Autodesk Inventor part; units mm, degrees
ref_plane "YZ Plane" through (0, 0, 0) normal (1, 0, 0) x (0, 1, 0)
ref_plane "XZ Plane" through (0, 0, 0) normal (0, 1, 0) x (-1, 0, 0)
ref_plane "XY Plane" through (0, 0, 0) normal (0, 0, 1) x (1, 0, 0)
sketch "Sketch1" plane through (0, 0, 0) normal (0, 1, 0) x (-1, 0, 0)
  line L0 (12.7, -15.875) -> (12.7, -12.7) construction
  line L1 (12.7, -12.7) -> (15.875, -10.8669) construction
  line L2 (15.875, -10.8669) -> (15.875, -7.9375) construction
  line L3 (15.875, -7.9375) -> (6.35, -7.9375) construction
  line L4 (6.35, -7.9375) -> (6.35, -3.175) construction
  line L5 (6.35, -3.175) -> (3.175, -3.175) construction
  line L6 (3.175, -3.175) -> (3.175, -6.35) construction
  line L7 (3.175, -6.35) -> (4.7625, -7.2665) construction
  line L8 (4.7625, -7.2665) -> (4.7625, -7.9375) construction
  line L9 (4.7625, -7.9375) -> (-4.7625, -7.9375) construction
  line L10 (-4.7625, -7.9375) -> (-4.7625, -7.2665) construction
  line L11 (-4.7625, -7.2665) -> (-3.175, -6.35) construction
  line L12 (-3.175, -6.35) -> (-3.175, -3.175) construction
  line L13 (-3.175, -3.175) -> (-6.35, -3.175) construction
  line L14 (-6.35, -3.175) -> (-6.35, -7.9375) construction
  line L15 (-6.35, -7.9375) -> (-15.875, -7.9375) construction
  line L16 (-15.875, -7.9375) -> (-15.875, -10.8669) construction
  line L17 (-15.875, -10.8669) -> (-12.7, -12.7) construction
  line L18 (-12.7, -12.7) -> (-12.7, -15.875) construction
  line L19 (-25.4, -15.875) -> (-12.7, -15.875) construction
  line L20 (-25.4, 0) -> (-25.4, -15.875) construction
  line L21 (25.4, 0) -> (-25.4, 0) construction
  line L22 (25.4, 0) -> (25.4, -15.875) construction
  line L23 (12.7, -15.875) -> (25.4, -15.875) construction
  line L24 (-12.3825, -15.875) -> (-12.3825, -12.5167)
  line L25 (-12.3825, -12.5167) -> (-15.5575, -10.6836)
  line L26 (-15.5575, -10.6836) -> (-15.5575, -8.255)
  line L27 (-15.5575, -8.255) -> (-6.0325, -8.255)
  line L28 (-6.0325, -8.255) -> (-6.0325, -3.4925) construction
  line L29 (-12.3825, -15.875) -> (0, -15.875)
  line L30 (0, -15.875) -> (0, -8.255)
  line L31 (-6.0325, -8.255) -> (0, -8.255)
  line L32 (0, -8.255) -> (0, -3.4925)
  line L33 (-3.175, -8.255) -> (-3.175, -5.08)
  line L34 (-3.175, -5.08) -> (-4.7625, -4.1635)
  line L35 (-4.7625, -4.1635) -> (-4.7625, -3.4925)
  line L36 (-6.0325, -3.4925) -> (-4.7625, -3.4925) construction
  line L37 (-4.7625, -3.4925) -> (0, -3.4925)
  point P0 (0, -7.9375)
  dimension "d1" = 0.3175
  dimension "d2" = 0.3175
  dimension "d3" = 0.3175
  dimension "d4" = 0.3175
  dimension "d5" = 0.3175
  dimension "d12" = 3.175
  dimension "d13" = 0.3175
  dimension "d14" = 30
extrude "Extrusion1" add sketch "Sketch1" along normal blind 76.2
extrude "Extrusion2" add sketch "Sketch1" against normal blind 38.1 contours L24 L25 L26 L27 L31 L30 L29
mirror "Mirror1" about plane through (0, 0, -8.255) normal (-1, 0, 0) of "Extrusion1", "Extrusion2"
sketch "Sketch2" plane through (0, -38.1, 0) normal (0, -1, 0) x (1, 0, 0)
  line L0 (12.3825, -15.875) -> (-12.3825, -15.875) construction
  line L1 (12.3825, -15.875) -> (12.3825, -12.5167) construction
  line L2 (12.3825, -12.5167) -> (15.5575, -10.6836) construction
  line L3 (15.5575, -10.6836) -> (15.5575, -8.255) construction
  line L4 (15.5575, -8.255) -> (-15.5575, -8.255) construction
  line L5 (-15.5575, -10.6836) -> (-15.5575, -8.255) construction
  line L6 (-12.3825, -12.5167) -> (-15.5575, -10.6836) construction
  line L7 (-12.3825, -15.875) -> (-12.3825, -12.5167) construction
  circle A0 centre (0, -16.6845) radius 5.08 construction
  line L8 (12.3825, -15.875) -> (-12.3825, -15.875) construction
  line L9 (6.2865, -15.875) -> (1.5875, -11.176)
  line L10 (1.5875, -11.176) -> (-1.5875, -11.176)
  line L11 (-1.5875, -11.176) -> (-6.2865, -15.875)
  line L12 (0, -11.176) -> (0, -15.875) construction
  line L13 (6.2865, -15.875) -> (-6.2865, -15.875)
  point P0 (0, 0)
  dimension "d15" = 10.16
  dimension "d16" = 4.699
  dimension "d17" = 45
  dimension "d18" = 3.175
extrude "Extrusion3" cut sketch "Sketch2" against normal through all
ref_plane "Work Plane1" through (0, -6.35, 0) normal (0, -1, 0) x (1, 0, 0)
sketch "Sketch3" plane through (0, -6.35, 0) normal (0, -1, 0) x (1, 0, 0)
  line L0 (-6.2865, -15.875) -> (-1.5875, -11.176) construction
  line L1 (-1.5875, -11.176) -> (1.5875, -11.176)
  line L2 (1.5875, -11.176) -> (6.2865, -15.875) construction
  line L3 (12.3825, -15.875) -> (6.2865, -15.875) construction
  line L4 (12.3825, -15.875) -> (12.3825, -12.5167)
  line L5 (12.3825, -12.5167) -> (15.5575, -10.6836)
  line L6 (15.5575, -10.6836) -> (15.5575, -8.255)
  line L7 (15.5575, -8.255) -> (-15.5575, -8.255) construction
  line L8 (-15.5575, -10.6836) -> (-15.5575, -8.255)
  line L9 (-12.3825, -12.5167) -> (-15.5575, -10.6836)
  line L10 (-12.3825, -15.875) -> (-12.3825, -12.5167)
  line L11 (-6.2865, -15.875) -> (-12.3825, -15.875)
  line L12 (12.3825, -15.875) -> (6.2865, -15.875) construction
  line L13 (11.3665, -15.875) -> (11.3665, -11.9301)
  line L14 (11.3665, -11.9301) -> (14.5415, -10.097) construction
  line L15 (14.5415, -10.097) -> (14.5415, -9.271) construction
  line L16 (14.5415, -9.271) -> (10.0965, -9.271) construction
  line L17 (0, -9.271) -> (0, -11.176) construction
  line L18 (1.5875, -11.176) -> (-1.5875, -11.176)
  line L19 (12.3825, -15.875) -> (11.3665, -15.875)
  line L20 (0, -9.271) -> (0, -8.255)
  line L21 (-3.175, -8.255) -> (3.175, -8.255) construction
  line L22 (15.5575, -8.255) -> (0, -8.255)
  line L23 (11.3665, -11.9301) -> (11.3665, -10.541)
  line L24 (11.3665, -10.541) -> (10.0965, -9.271)
  line L25 (10.0965, -9.271) -> (0, -9.271)
  point P0 (0, 0)
  dimension "d22" = 1.016
  dimension "d23" = 1.016
  dimension "d24" = 1.016
  dimension "d25" = 1.016
  dimension "d26" = 45
  dimension "d27" = 1.27
extrude "Extrusion4" cut sketch "Sketch3" against normal blind 3.175
ref_plane "Work Plane2" through (0, 44.45, 0) normal (0, 1, 0) x (1, 0, 0)
sketch "Sketch4" plane through (0, 44.45, 0) normal (0, 1, 0) x (1, 0, 0)
  line L0 (-1.5875, 11.176) -> (-6.2865, 15.875) construction
  line L1 (-6.2865, 15.875) -> (-12.3825, 15.875) construction
  line L2 (-12.3825, 12.5167) -> (-12.3825, 15.875) construction
  line L3 (-15.5575, 10.6836) -> (-12.3825, 12.5167) construction
  line L4 (-15.5575, 8.255) -> (-15.5575, 10.6836) construction
  line L5 (-3.175, 8.255) -> (-15.5575, 8.255) construction
  line L6 (-3.175, 5.08) -> (-3.175, 8.255) construction
  line L7 (-4.7625, 4.1635) -> (-3.175, 5.08) construction
  line L8 (-4.7625, 3.4925) -> (-4.7625, 4.1635) construction
  line L9 (4.7625, 3.4925) -> (-4.7625, 3.4925) construction
  line L10 (4.7625, 3.4925) -> (4.7625, 4.1635)
  line L11 (4.7625, 4.1635) -> (3.175, 5.08)
  line L12 (3.175, 5.08) -> (3.175, 8.255)
  line L13 (3.175, 8.255) -> (15.5575, 8.255)
  line L14 (15.5575, 8.255) -> (15.5575, 10.6836)
  line L15 (15.5575, 10.6836) -> (12.3825, 12.5167)
  line L16 (12.3825, 12.5167) -> (12.3825, 15.875)
  line L17 (12.3825, 15.875) -> (6.2865, 15.875) construction
  line L18 (6.2865, 15.875) -> (1.5875, 11.176) construction
  line L19 (1.5875, 11.176) -> (-1.5875, 11.176) construction
  line L20 (12.3825, 15.875) -> (6.2865, 15.875) construction
  line L21 (11.3665, 15.875) -> (11.3665, 10.541)
  line L22 (11.3665, 10.541) -> (10.0965, 9.271)
  line L23 (10.0965, 9.271) -> (0, 9.271)
  line L24 (0, 9.271) -> (0, 3.4925)
  line L25 (4.7625, 3.4925) -> (-4.7625, 3.4925) construction
  line L26 (12.3825, 15.875) -> (11.3665, 15.875)
  line L27 (4.7625, 3.4925) -> (0, 3.4925)
  point P0 (0, 0)
  dimension "d37" = 1.016
  dimension "d38" = 45
  dimension "d39" = 1.016
  dimension "d40" = 1.27
extrude "Extrusion5" cut sketch "Sketch4" against normal blind 3.175
mirror "Mirror2" about plane through (0, 0, 0) normal (1, 0, 0) of "Extrusion4", "Extrusion5"
equation "\"d2\" = d1"
equation "\"d3\" = d1"
equation "\"d4\" = d1"
equation "\"d5\" = d1"
equation "\"d13\" = d1"
equation "\"d23\" = d22"
equation "\"d24\" = d22"
equation "\"d25\" = d22"
equation "\"d37\" = d22"
equation "\"d39\" = d22"
properties part number "Holder_Slide" material "ABS Plastic"
CAD build for the part. Positions are in the model's coordinates, mm. A direction names the side the tool comes from. Coordinates: 2 decimals unless noted, no trailing zeros. Order: outer loops, then holes, each group sorted by start corner. A loop starts at its lowest first (then second) coordinate and runs counter-clockwise, first axis right, second up.
Item 1: Band-saw the part on C-C on y = 68. List the corners of the cut face in (x, z) (1 decimal).
Check sheet entries:
outline: (-15.6, -10.7) - (-12.4, -12.5) - (-12.4, -15.9) - (-6.3, -15.9) - (-1.6, -11.2) - (1.6, -11.2) - (6.3, -15.9) - (12.4, -15.9) - (12.4, -12.5) - (15.6, -10.7) - (15.6, -8.3) - (3.2, -8.3) - (3.2, -5.1) - (4.8, -4.2) - (4.8, -3.5) - (-4.8, -3.5) - (-4.8, -4.2) - (-3.2, -5.1) - (-3.2, -8.3) - (-15.6, -8.3) - close
Item 2: 3-axis set-ups, long thin cutter, end or side, ignore diameter. For faces 1 (the face through (-11.366, 43, -13)), 2 (the face through (11.366, 43, -13)), 3 (the face through (0, -6.35, -9)): which of +Z, -Z, +X, -X, +Y, -Y reach the whole face in a straight line?
Check sheet entries:
face 1: +Z, -Z, -X
face 2: +Z, -Z, +X
face 3: +Z
Item 3: Drill centre lines: L1, parallel to Y at x = -0.5, z = -8 (3 decimals); L2, parallel to Y at x = 12.5, z = -11.25 (3 decimals); L3, parallel to X at y = 3, z = -12.75. Where is each one in solid material? Low to high.
Check sheet entries:
L1: y = 0 to 41.275, 44.45 to 76.2
L2: y = -38.1 to -6.35, -3.175 to 41.275, 44.45 to 76.2
L3: x = -12.38 to -3.16, 3.16 to 12.38
Item 4: Band-saw the part on A-A on x = 13.5. Give the number of separate pieces and of enclosed holes in the cut face, plus the area to 3 significant figures.
Check sheet entries:
separate pieces: 3
enclosed holes: 0
area: 390 mm2
Item 5: Pin check, flat tips, straight feed: pin 1 Ø2 at (y, z) = (63, -5) entering from +X; pin 2 Ø2.5 at (y, z) = (10, -14.5) entering from -X; pin 3 Ø1 at (y, z) = (62, -7) entering from +X (3 decimals). Stop position of each tip, or through.
Check sheet entries:
pin 1: stops at x = 4.76
pin 2: stops at x = -12.38
pin 3: stops at x = 3.175
